Read the model definition and answer for the solid it produces. Units are mm, in the model's axes. Coordinates: 2 decimals unless noted, no trailing zeros. Loops run counter-clockwise (first coordinate to the right, second up) from the corner with the lowest first, then second, coordinate; pieces in that order, holes last. Notation, with made-up numbers: M 80.5,82 L 95.5,82 A19 ccw 95.5,96 Z; hole C 32,81 d8. An arc over 180 degrees is marked long. One line per item, written item: value. Start each with the question number.
1. Flat-ended cylindrical pins translate along their axes: pin 1 (12 mm diameter, centred on x = -8, y = 8, fed in from +Z); pin 2 (2 mm diameter, centred on y = -36, z = 6.5, fed in from -X) (3 decimals); pin 3 (2 mm diameter, centred on x = 1.5, z = 6, fed in from -Y). Find the tip coordinate at first contact, or state that the pin passes through.
2. Consider probe 1 along X at (y, z) = (32.5, 5.5); probe 2 along Y at (x, z) = (-10.5, 3); probe 3 along Y at (x, z) = (8.5, 2.25). Determine where each line is inside the solid, lowest interval first.
3. The part is cut by section C-C (x = 2). State how many separate pieces and enclosed holes the cut face has, then the cut area to 3 significant figures.
4. The part is cut by section B-B (z = 5). Write down the section's boundary in (x, y).
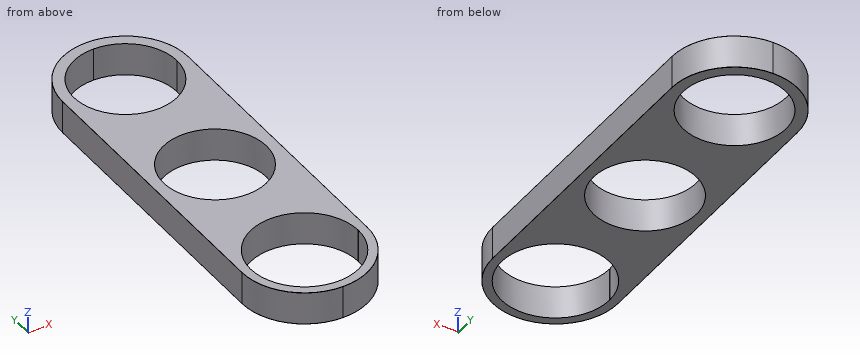
```python
from build123d import *

# Parameters (mm, degrees)
F1_DEPTH = 7.3
F2_R     = 0.0241421356


with BuildPart() as f1:
    # F0 (on Top) → F1 (new body)
    with BuildSketch(Plane.XY):
        with BuildLine():
            ThreePointArc((14, 32.5), (9.8994949366, 42.3994949366), (0, 46.5))
            ThreePointArc((0, 46.5), (-9.8994949366, 42.3994949366), (-14, 32.5))
            Line((-14, 32.5), (-14, -32.5))
            Line((-14, -32.5), (-12.0277635282, -32.5))
            ThreePointArc((-12.0277635282, -32.5), (-12.0273670809, -32.4023445279), (-12.0261777652, -32.3046954935))
            ThreePointArc((-12.0261777652, -32.3046954935), (0, -20.4722364718), (12.0261777652, -32.3046954935))
            ThreePointArc((12.0261777652, -32.3046954935), (12.0273670809, -32.4023445279), (12.0277635282, -32.5))
            ThreePointArc((12.0277635282, -32.5), (8.5049131533, -41.0049131533), (0, -44.5277635282))
            Line((0, -44.5277635282), (0, -46.5))
            ThreePointArc((0, -46.5), (9.8994949366, -42.3994949366), (14, -32.5))
            Line((14, -32.5), (14, 32.5))
        make_face()
        with BuildLine():
            ThreePointArc((-11.5, 0), (0, 11.5), (11.5, 0))
            ThreePointArc((11.5, 0), (0, -11.5), (-11.5, 0))
        make_face(mode=Mode.SUBTRACT)
        with BuildLine():
            ThreePointArc((11.5, 32.5), (-8.1317279836, 24.3682720164), (0, 44))
            ThreePointArc((0, 44), (8.1317279836, 40.6317279836), (11.5, 32.5))
        make_face(mode=Mode.SUBTRACT)
        with BuildLine():
            Line((-12.0277635282, -32.5), (-14, -32.5))
            ThreePointArc((-14, -32.5), (-9.8994949366, -42.3994949366), (0, -46.5))
            Line((0, -46.5), (0, -44.5277635282))
            ThreePointArc((0, -44.5277635282), (-8.5049131533, -41.0049131533), (-12.0277635282, -32.5))
        make_face()
    extrude(amount=F1_DEPTH)

    # F2
    f2_edges = [f1.edges().sort_by_distance(p)[0] for p in [
        (0, 46.5, 7.3),
        (-14, 0, 7.3),
        (0, -46.5, 7.3),
        (14, 0, 7.3),
        (0, 46.5, 0),
        (14, 0, 0),
        (-14, 0, 0),
        (0, -46.5, 0),
    ]]
    fillet(f2_edges, radius=F2_R)


solid = f1.part
```
Answer block:
1. pin 1: stops at z = 7.3
1. pin 2: stops at x = -13.775
1. pin 3: stops at y = -46.49
2. probe 1: x = -14 to -11.5, 11.5 to 14
2. probe 2: y = -41.76 to -38.37, -26.63 to -4.69, 4.69 to 27.81, 37.19 to 41.76
2. probe 3: y = -43.62 to -41.01, -23.99 to -7.75, 7.75 to 24.75, 40.25 to 43.62
3. separate pieces: 4
3. enclosed holes: 0
3. area: 173 mm2
4. outline: M -14,-32.5 A14 ccw 14,-32.5 L 14,32.5 A14 ccw -14,32.5 Z; hole C 0,-32.5 d24.06; hole C 0,0 d23; hole C 0,32.5 d23
